CAD build for the part. Positions are in the model's coordinates, mm. A direction names the side the tool comes from. Round coordinates to 2 decimals unless told otherwise and drop trailing zeros. Order: outer loops, then holes, each group sorted by start corner. A loop starts at its lowest first (then second) coordinate and runs counter-clockwise, first axis right, second up. Notation, with made-up numbers: M 36,81.5 L 69,81.5 A22 cw 69,93.5 Z; hole C 55.5,31.5 d1. An arc over 180 degrees is marked long. Put each result on its own line as item: value.
```python
from build123d import *

# Parameters (mm, degrees)
SKETCH1_W                                           = 50
SKETCH1_H                                           = 50
SKETCH1_R                                           = 20.85
BOSS_EXTRUDE1_DEPTH                                 = 10
SKETCH2_W                                           = 3.5
SKETCH2_H                                           = 12.12353247
CUT_EXTRUDE1_DEPTH                                  = 10
CHAMFER1_SIZE                                       = 2
FILLET1_R                                           = 1
F_5_2_5_2_DIAMETER_HOLE1_D                          = 5.2
F_5_2_5_2_DIAMETER_HOLE1_DEPTH                      = 10
F_5_2_5_2_DIAMETER_HOLE1_TIP                        = 1.562237609
CBORE_FOR_M5_HEX_SOCKET_HEAD_CAP_SCREW1_D           = 5.5
CBORE_FOR_M5_HEX_SOCKET_HEAD_CAP_SCREW1_CBORE_D     = 9
CBORE_FOR_M5_HEX_SOCKET_HEAD_CAP_SCREW1_CBORE_DEPTH = 6


with BuildPart() as part:
    # Sketch1 → Boss-Extrude1 (new body)
    with BuildSketch(Plane(origin=(0, 0, 0), x_dir=(1, 0, 0), z_dir=(0, 1, 0))):
        Rectangle(SKETCH1_W, SKETCH1_H)
        Circle(SKETCH1_R, mode=Mode.SUBTRACT)
    extrude(amount=BOSS_EXTRUDE1_DEPTH)

    # Sketch2 → Cut-Extrude1 (cut)
    with BuildSketch(Plane(origin=(0, 10, 0), x_dir=(1, 0, 0), z_dir=(0, 1, 0))):
        with Locations((0, -25)):
            Rectangle(SKETCH2_W, SKETCH2_H)
    extrude(amount=-CUT_EXTRUDE1_DEPTH, mode=Mode.SUBTRACT)

    # Chamfer1
    chamfer1_edges = [part.edges().sort_by_distance(p)[0] for p in [
        (25, 5, 25),
        (-25, 5, 25),
        (-25, 5, -25),
        (25, 5, -25),
    ]]
    chamfer(chamfer1_edges, length=CHAMFER1_SIZE)

    # Fillet1
    fillet1_edges = [part.edges().sort_by_distance(p)[0] for p in [
        (-1.75, 5, 20.776428952),
        (1.75, 5, 20.776428952),
        (1.75, 5, 25),
        (-1.75, 5, 25),
        (-25, 5, 23),
        (-25, 5, -23),
        (23, 5, -25),
        (-23, 5, -25),
        (-23, 5, 25),
        (25, 5, 23),
        (25, 5, -23),
        (23, 5, 25),
    ]]
    fillet(fillet1_edges, radius=FILLET1_R)

    # Ø5.2 (5.2) Diameter Hole1
    with Locations(Plane(origin=(-20, 10, -20), x_dir=(0, 0, 1), z_dir=(0, 1, 0))):
        with Locations((0, 0), (0, 40), (40, 40), (40, 0)):
            Hole(F_5_2_5_2_DIAMETER_HOLE1_D / 2, depth=F_5_2_5_2_DIAMETER_HOLE1_DEPTH)
            with Locations((0, 0, -(F_5_2_5_2_DIAMETER_HOLE1_DEPTH + F_5_2_5_2_DIAMETER_HOLE1_TIP / 2))):  # 118° drill point
                Cone(0, F_5_2_5_2_DIAMETER_HOLE1_D / 2, F_5_2_5_2_DIAMETER_HOLE1_TIP, mode=Mode.SUBTRACT)

    # CBORE for M5 Hex Socket Head Cap Screw1 (through all)
    with Locations(Plane(origin=(-20, 10, -20), x_dir=(0, 0, 1), z_dir=(0, 1, 0))):
        with Locations((0, 0), (40, 0), (40, 40), (0, 40)):
            CounterBoreHole(CBORE_FOR_M5_HEX_SOCKET_HEAD_CAP_SCREW1_D / 2, CBORE_FOR_M5_HEX_SOCKET_HEAD_CAP_SCREW1_CBORE_D / 2, CBORE_FOR_M5_HEX_SOCKET_HEAD_CAP_SCREW1_CBORE_DEPTH)


solid = part.part
```
Item 1: Band-saw the part on B-B on z = 0. Give the cut face in (x, y), and give its area (3 significant figures).
Answers below:
outline: M -25,0 L -20.85,0 L -20.85,10 L -25,10 Z; M 20.85,0 L 25,0 L 25,10 L 20.85,10 Z
area: 83.0 mm²
Item 2: Band-saw the part on C-C on x = 20. Give the cut face in (y, z), and give its area (3 significant figures).
Answers below:
outline: M 0,-25 L 10,-25 L 10,-24.5 L 4,-24.5 L 4,-22.75 L 0,-22.75 Z; M 0,-17.25 L 4,-17.25 L 4,-15.5 L 10,-15.5 L 10,-5.89 L 0,-5.89 Z; M 0,5.89 L 10,5.89 L 10,15.5 L 4,15.5 L 4,17.25 L 0,17.25 Z; M 0,22.75 L 4,22.75 L 4,24.5 L 10,24.5 L 10,25 L 0,25 Z
area: 230 mm²
Item 3: Band-saw the part on D-D on z = 20. Give the cut face in (x, y), and give its area (3 significant figures).
Answers below:
outline: M -25,0 L -22.75,0 L -22.75,4 L -24.5,4 L -24.5,10 L -25,10 Z; M -17.25,0 L -5.89,0 L -5.89,10 L -15.5,10 L -15.5,4 L -17.25,4 Z; M 5.89,0 L 17.25,0 L 17.25,4 L 15.5,4 L 15.5,10 L 5.89,10 Z; M 22.75,0 L 25,0 L 25,10 L 24.5,10 L 24.5,4 L 22.75,4 Z
area: 230 mm²
Item 4: Band-saw the part on A-A on y = 1.25. Give the cut face in (x, z), and give its area (3 significant figures).
Answers below:
outline: M -25,-22.59 A1 ccw -24.71,-23.29 L -23.29,-24.71 A1 ccw -22.59,-25 L 22.59,-25 A1 ccw 23.29,-24.71 L 24.71,-23.29 A1 ccw 25,-22.59 L 25,22.59 A1 ccw 24.71,23.29 L 23.29,24.71 A1 ccw 22.59,25 L 2.75,25 A1 ccw 1.75,24 L 1.75,21.68 A1 ccw 2.62,20.68 A20.85 cw long -2.62,20.68 A1 ccw -1.75,21.68 L -1.75,24 A1 ccw -2.75,25 L -22.59,25 A1 ccw -23.29,24.71 L -24.71,23.29 A1 ccw -25,22.59 Z; hole C -20,-20 d5.5; hole C -20,20 d5.5; hole C 20,-20 d5.5; hole C 20,20 d5.5
area: 1,020 mm²
Item 5: Probe line 1 along X through (y, z) = (1.25, -22.5); line 2 along Z through (x, y) = (-19, 9.25); line 3 along Y through (x, z) = (-17, 22). List the from-to ranges inside material, lowest first. Write a range as [from, to].
Answers below:
line 1: [-25, -21.15], [-18.85, 18.85], [21.15, 25]
line 2: [-25, -24.39], [-15.61, -8.59], [8.59, 15.61], [24.39, 25]
line 3: [0, 4]
Item 6: Tool access for faces 1 (the flat face through (25, 5, 0)), 2 (the flat face through (-1.75, 5, 23)), 3 (the flat face through (-23, 4, -20)): list every direction of +Z, -Z, +X, -X, +Y, -Y with a clear straight run to the whole face (end or side of a thin tool).
Answers below:
face 1: +Z, -Z, +X, +Y, -Y
face 2: +Z, +Y, -Y
face 3: +Y
Item 7: Pin check, flat tips, straight feed: P1, Ø14.5, axis at x = 20, z = 20, coming from the -Y side; P2, Ø2.5, axis at x = -18.5, z = -18.5, coming from the +Y side. Stop position of each tip, or through.
Answers below:
P1: y = 0
P2: y = 4
Item 8: Mould opens along X. For faces 4 (the flat face through (0, 0, -23)), 5 (the flat face through (24, 5, 24)), 6 (the cylindrical face through (-19.879, 1.972, 22.747)) say: pulls with the +X half, pulls with the -X half, needs draft (parallel to the pull), parting line crosses it, or undercut.
Answers below:
face 4: needs draft
face 5: pulls with the +X half
face 6: undercut
